For this review, take the finished solid that the model builds, in its own axes (mm). A direction names the side the tool comes from. Coordinates: 2 decimals unless noted, no trailing zeros. Loops run counter-clockwise (first coordinate to the right, second up) from the corner with the lowest first, then second, coordinate; pieces in that order, holes last. Notation, with made-up numbers: (75, 25.25) - (110, 25.25) arc R14 ccw to (110, 46.25) - close; hole circle Ø10 at (-27.5, -39). An arc over 180 degrees is marked (long way). Use one line per item in the form item = value. Start each with the question number.
1. To check wall thickness, follow probe 1 along Z at (x, y) = (20, 4.5); probe 2 along X at (y, z) = (0.25, -8); probe 3 along Z at (x, y) = (7, 0.5). State the ranges of each line that lie inside material, in increasing order.
2. Draft analysis for pull direction Z (two halves, no side actions). For faces 3 (the face through (0, 0, -22)), 4 (the face through (9.091, 0.085, -9.293)), 5 (the face through (24.064, -4.261, -5.496)), state which applies: +Z half, -Z half, draft (parallel to the pull), parting line (faces both ways), or undercut.
3. Add section C-C on y = 8.75. Give the boundary of the cut face in (x, z), and give its area (3 significant figures).
4. Add section A-A on y = 4.5. Give the boundary of the cut face in (x, z), and give its area (3 significant figures).
5. Machinability: for faces 1 (the face through (8.37, -4.26, -17.91)), 2 (the face through (15, -12.5, -16)), which of the approach directions +Z, -Z, +X, -X, +Y, -Y give a long, thin tool a straight path to every point of the face, cutting with its end or side? Answer none if there is none.
6. For pin 1 Ø6 at (x, z) = (7.5, -7.5) entering from -Y; pin 2 Ø5 at (x, y) = (7.5, -9) entering from -Z; pin 3 Ø3 at (y, z) = (-4.5, -9.5) entering from +X; pin 4 Ø4 at (x, z) = (6.8, -20.92) entering from -Y, all flat-tipped, find the tip position at first contact; note any pin that passes through.
7. Add section B-B on y = -3.25. Give the boundary of the cut face in (x, z).
```python
from build123d import *

# Parameters (mm, degrees)
AUFSATZ_LINEAR_AUSTRAGEN1_DEPTH = 12.5
M8_GEWINDEBOHRUNG1_D            = 6.8
M8_GEWINDEBOHRUNG1_DEPTH        = 16.25
M8_GEWINDEBOHRUNG1_TIP          = 2.042926105


with BuildPart() as part:
    # Skizze1 → Aufsatz-Linear austragen1 (new, symmetric)
    with BuildSketch(Plane(origin=(0, 0, 0), x_dir=(1, 0, 0), z_dir=(0, 1, 0))):
        with BuildLine():
            Line((0, 31), (0, 13))
            ThreePointArc((0, 13), (9.192388155, 9.192388155), (13, 0))
            Line((13, 0), (31, 0))
            ThreePointArc((31, 0), (21.920310217, 21.920310217), (0, 31))
        make_face()
    extrude(amount=AUFSATZ_LINEAR_AUSTRAGEN1_DEPTH, both=True)

    # Schnitt-Austragung1: sweep along a curve in space
    with BuildLine() as schnitt_austragung1_path:
        ThreePointArc((31, 12.5, 0), (21.920310217, 12.5, -21.920310217), (0, 12.5, -31))
    # Skizze2 → Schnitt-Austragung1 (sweep, cut)
    with BuildSketch(Plane.XY):
        Polygon((13, 12.5), (31, 12.5), (31, 7.5), (13, 12.323085464), align=None)
    sweep(path=schnitt_austragung1_path.line, mode=Mode.SUBTRACT)

    # M8 Gewindebohrung1
    with Locations(Plane(origin=(0, -12.5, 0), x_dir=(-1, 0, 0), z_dir=(0, -1, 0))):
        with Locations((-6.798373876, 20.923243358), (-20.923243358, 6.798373876)):
            Hole(M8_GEWINDEBOHRUNG1_D / 2, depth=M8_GEWINDEBOHRUNG1_DEPTH)
            with Locations((0, 0, -(M8_GEWINDEBOHRUNG1_DEPTH + M8_GEWINDEBOHRUNG1_TIP / 2))):  # 118° drill point
                Cone(0, M8_GEWINDEBOHRUNG1_D / 2, M8_GEWINDEBOHRUNG1_TIP, mode=Mode.SUBTRACT)


solid = part.part
```
Conclusion:
q1.probe_1 = -23.69 to -8.74, -4.85 to 0
q1.probe_2 = 10.25 to 17.74, 24.1 to 29.95
q1.probe_3 = -30.2 to -24.32, -17.53 to -10.95
q2.face_3 = draft
q2.face_4 = +Z half
q2.face_5 = undercut
q3.outline = (0, -26.33) arc R26.33 ccw to (26.33, 0) - (13, 0) arc R13 cw to (0, -13) - close
q3.area = 412 mm^2
q4.outline = (0, -31) arc R31 ccw to (31, 0) - (13, 0) arc R13 cw to (0, -13) - close; hole circle Ø4.3 at (6.8, -20.92); hole circle Ø4.3 at (20.92, -6.8)
q4.area = 593 mm^2
q5.face_1 = -Y
q5.face_2 = +Z, -Z, +X, -X, -Y
q6.pin_1 = -12.5
q6.pin_2 = -30.59
q6.pin_3 = 29.95
q6.pin_4 = 4.59
q7.outline = (0, -31) arc R31 ccw to (31, 0) - (13, 0) arc R13 cw to (0, -13) - close; hole circle Ø6.8 at (6.8, -20.92); hole circle Ø6.8 at (20.92, -6.8)
